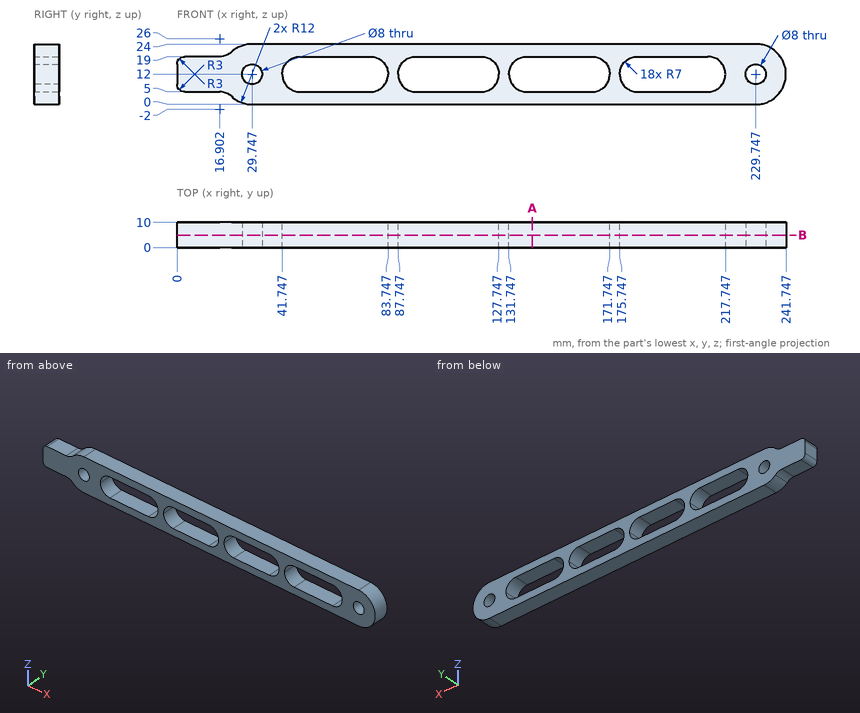
Design review of the part shown in the three views and the two pictorial views. Dimensions are in mm from the part's minimum x, y and z. Round coordinates to 2 decimals unless told otherwise and drop trailing zeros. Write each loop counter-clockwise with the first axis right and the second up, starting at its lowest first coordinate (ties: lowest second). Pieces come first, ordered by that corner, then holes. Notation, with made-up numbers: (-33.75, 19) -> (8.25, 19) arc R20 ccw to (8.25, 57) -> close; hole circle Ø9 at (2, 48.5). An arc over 180 degrees is marked (long way). Answer as a JSON object with one key per item and string values.
1. We need section A-A on x = 141. State the section outline as (y, z) points.
Results found:
{"outline": "(0, 0) -> (10, 0) -> (10, 5) -> (0, 5) -> close; (0, 19) -> (10, 19) -> (10, 24) -> (0, 24) -> close"}
2. Clearance check with flat-ended pins moving along their axes: pin 1 (4 mm diameter, centred on y = 5, z = 18.5, fed in from +X); pin 2 (3 mm diameter, centred on x = 6.5, y = 4, fed in from +Z). State where each tip first meets the part, or that it passes through.
Results found:
{"pin 1": "stops at x = 240.87", "pin 2": "stops at z = 19"}
3. We need section B-B on y = 5. State how many separate pieces and enclosed holes the cut face has, and give its area (3 significant figures).
Results found:
{"separate pieces": "1", "enclosed holes": "6", "area": "3,280 mm^2"}
4. To check wall thickness, follow line 1 along Z through (x, y) = (145, 8); line 2 along Z through (x, y) = (216.5, 1.25) (1 decimal); line 3 along X through (y, z) = (7.75, 6.5) (1 decimal). State the ranges of each line that lie inside material, in increasing order.
Results found:
{"line 1": "z = 0 to 5, 19 to 24", "line 2": "z = 0 to 8, 16 to 24", "line 3": "x = 0.4 to 44.4, 81.1 to 90.4, 125.1 to 134.4, 169.1 to 178.4, 215.1 to 240.4"}
